from build123d import *

# Parameters (mm, degrees)
EXTRUDE_5_DEPTH     = 5
EXTRUDE_5_DRAFT     = 3
SKETCH_1_9_R        = 3.75
CUT_EXTRUDE_1_DEPTH = 71.129382412


with BuildPart() as part:
    # ｽｹｯﾁ1 → ﾎﾞｽ - 押し出し5 (with draft: the straight prism first)
    with BuildSketch(Plane.XY):
        with BuildLine():
            ThreePointArc((-59.25, -31.5), (-57.785533906, -35.035533906), (-54.25, -36.5))
            Line((-54.25, -36.5), (54.25, -36.5))
            ThreePointArc((54.25, -36.5), (57.785533906, -35.035533906), (59.25, -31.5))
            Line((59.25, -31.5), (59.25, 31.5))
            ThreePointArc((59.25, 31.5), (57.785533906, 35.035533906), (54.25, 36.5))
            Line((54.25, 36.5), (-54.25, 36.5))
            ThreePointArc((-54.25, 36.5), (-57.785533906, 35.035533906), (-59.25, 31.5))
            Line((-59.25, 31.5), (-59.25, -31.5))
        make_face()
        with BuildLine():
            Line((-54.25, 32.5), (-47.4, 32.5))
            Line((-47.4, 32.5), (-47.4, 25))
            ThreePointArc((-47.4, 25), (-42, 19.6), (-36.6, 25))
            Line((-36.6, 25), (-36.6, 32.5))
            Line((-36.6, 32.5), (36.6, 32.5))
            Line((36.6, 32.5), (36.6, 25))
            ThreePointArc((36.6, 25), (42, 19.6), (47.4, 25))
            Line((47.4, 25), (47.4, 32.5))
            Line((47.4, 32.5), (54.25, 32.5))
            ThreePointArc((54.25, 32.5), (54.957106781, 32.207106781), (55.25, 31.5))
            Line((55.25, 31.5), (55.25, -31.5))
            ThreePointArc((55.25, -31.5), (54.957106781, -32.207106781), (54.25, -32.5))
            Line((54.25, -32.5), (47.4, -32.5))
            Line((47.4, -32.5), (47.4, -25))
            ThreePointArc((47.4, -25), (42, -19.6), (36.6, -25))
            Line((36.6, -25), (36.6, -32.5))
            Line((36.6, -32.5), (-36.6, -32.5))
            Line((-36.6, -32.5), (-36.6, -25))
            ThreePointArc((-36.6, -25), (-42, -19.6), (-47.4, -25))
            Line((-47.4, -25), (-47.4, -32.5))
            Line((-47.4, -32.5), (-54.25, -32.5))
            ThreePointArc((-54.25, -32.5), (-54.957106781, -32.207106781), (-55.25, -31.5))
            Line((-55.25, -31.5), (-55.25, 31.5))
            ThreePointArc((-55.25, 31.5), (-54.957106781, 32.207106781), (-54.25, 32.5))
        make_face(mode=Mode.SUBTRACT)
    extrude(amount=-EXTRUDE_5_DEPTH)
    # ﾎﾞｽ - 押し出し5: the draft: its side faces are tilted about the plane it starts from
    extrude_5_sides = [part.faces().sort_by_distance(p)[0] for p in [
        (-57.785533906, -35.035533906, -2.5),
        (0, -36.5, -2.5),
        (57.785533906, -35.035533906, -2.5),
        (59.25, 0, -2.5),
        (57.785533906, 35.035533906, -2.5),
        (0, 36.5, -2.5),
        (-57.785533906, 35.035533906, -2.5),
        (-59.25, 0, -2.5),
        (-50.825, 32.5, -2.5),
        (-47.4, 28.75, -2.5),
        (-42, 19.6, -2.5),
        (-36.6, 28.75, -2.5),
        (0, 32.5, -2.5),
        (36.6, 28.75, -2.5),
        (42, 19.6, -2.5),
        (47.4, 28.75, -2.5),
        (50.825, 32.5, -2.5),
        (54.957106781, 32.207106781, -2.5),
        (55.25, 0, -2.5),
        (54.957106781, -32.207106781, -2.5),
        (50.825, -32.5, -2.5),
        (47.4, -28.75, -2.5),
        (42, -19.6, -2.5),
        (36.6, -28.75, -2.5),
        (0, -32.5, -2.5),
        (-36.6, -28.75, -2.5),
        (-42, -19.6, -2.5),
        (-47.4, -28.75, -2.5),
        (-50.825, -32.5, -2.5),
        (-54.957106781, -32.207106781, -2.5),
        (-55.25, 0, -2.5),
        (-54.957106781, 32.207106781, -2.5),
    ]]
    draft(extrude_5_sides, Plane.XY, EXTRUDE_5_DRAFT)

    # ｽｹｯﾁ1<9> → ｶｯﾄ - 押し出し1 (cut, through all)
    with BuildSketch(Plane.XY):
        with Locations((-42, 25)):
            Circle(SKETCH_1_9_R)
        with Locations((-42, -25)):
            Circle(SKETCH_1_9_R)
        with Locations((42, -25)):
            Circle(SKETCH_1_9_R)
        with Locations((42, 25)):
            Circle(SKETCH_1_9_R)
    extrude(amount=-CUT_EXTRUDE_1_DEPTH, mode=Mode.SUBTRACT)


solid = part.part
For this review, take the finished solid that the model builds, in its own axes (mm). A direction names the side the tool comes from. Coordinates: 2 decimals unless noted, no trailing zeros. Loops run counter-clockwise (first coordinate to the right, second up) from the corner with the lowest first, then second, coordinate; pieces in that order, holes last. Notation, with made-up numbers: (-40, 24) - (-8, 24) arc R20 cw to (-8, 61) - close; hole circle Ø9 at (59.25, -35). An arc over 180 degrees is marked (long way). Use a Markdown table: item, result. Add a question column.
Item 1: Mouldability with a two-part tool opening along Y and no side actions: class faces 3 (the face through (-55.12, -0.44, -2.47)), 4 (the face through (0, -33, -5)), 5 (the face through (-57.917, -35.087, -2.465)) as pulls with the +Y half, pulls with the -Y half, needs draft (parallel to the pull), parting line crosses it, or undercut.
Item 2: For line 1 (Y direction, x = -42, z = -2.8); line 2 (Y direction, x = -42, z = -3.5); line 3 (X direction, y = 21, z = -2.7), list the stretches that pass through material, from the lowest coordinate up.
Item 3: We need section B-B (y = -5). Give the boundary of the cut face in (x, z), and give its area (3 significant figures).
Item 4: We need section A-A (x = 42). Give the boundary of the cut face in (y, z), and give its area (3 significant figures).
Item 5: Insertion check: pin 1 Ø7 at (x, y) = (-42, 25) entering from -Z; pin 2 Ø1.5 at (y, z) = (-19, -4) entering from +X. Each pin has a flat end and moves straight along its axis. Give the tip position at first contact, or say it passes through.
Item 6: We need section D-D (z = -2.5). Give the number of separate pieces and of enclosed holes in the cut face, and give its area (3 significant figures).
Item 7: We need section C-C (x = 2). Give the boundary of the cut face in (y, z).
Item 8: Tool access review of faces 1 (the face through (36.47, 28.8, -2.47)), 2 (the face through (39.024, -27.282, -2.465)): name each direction out of +Z, -Z, +X, -X, +Y, -Y from which nothing blocks a thin tool from reaching the whole face with its end or side.
Results list:
| question | item | result |
|---|---|---|
| 1 | face 3 | undercut |
| 1 | face 4 | needs draft |
| 1 | face 5 | pulls with the -Y half |
| 2 | line 1 | y = -36.65 to -28.75, -21.25 to -19.45, 19.45 to 21.25, 28.75 to 36.65 |
| 2 | line 2 | y = -36.68 to -28.75, -21.25 to -19.42, 19.42 to 21.25, 28.75 to 36.68 |
| 2 | line 3 | x = -59.39 to -55.11, -45.84 to -38.16, 38.16 to 45.84, 55.11 to 59.39 |
| 3 | outline | (-59.51, -5) - (-54.99, -5) - (-55.25, 0) - (-59.25, 0) - close; (54.99, -5) - (59.51, -5) - (59.25, 0) - (55.25, 0) - close |
| 3 | area | 42.6 mm^2 |
| 4 | outline | (-36.76, -5) - (-28.75, -5) - (-28.75, 0) - (-36.5, 0) - close; (-21.25, -5) - (-19.34, -5) - (-19.6, 0) - (-21.25, 0) - close; (19.34, -5) - (21.25, -5) - (21.25, 0) - (19.6, 0) - close; (28.75, -5) - (36.76, -5) - (36.5, 0) - (28.75, 0) - close |
| 4 | area | 96.6 mm^2 |
| 5 | pin 1 | passes through |
| 5 | pin 2 | stops at x = 59.5 |
| 6 | separate pieces | 1 |
| 6 | enclosed holes | 5 |
| 6 | area | 1,880 mm^2 |
| 7 | outline | (-36.76, -5) - (-32.24, -5) - (-32.5, 0) - (-36.5, 0) - close; (32.24, -5) - (36.76, -5) - (36.5, 0) - (32.5, 0) - close |
| 8 | face 1 | +Z |
| 8 | face 2 | +Z, -Z |
